Answer from the drawing. Dimensions are ordinates in mm from the lowest x, y and z of the part. Coordinates: 2 decimals unless noted, no trailing zeros. Order: outer loops, then holes, each group sorted by start corner. A loop starts at its lowest first (then second) coordinate and runs counter-clockwise, first axis right, second up. Notation, with made-up numbers: M 2.5,54 L 13.5,54 A32 cw 13.5,92 Z; hole C -0.5,-18 d7. An arc over 180 degrees is marked long. Use a Markdown table: item, result.
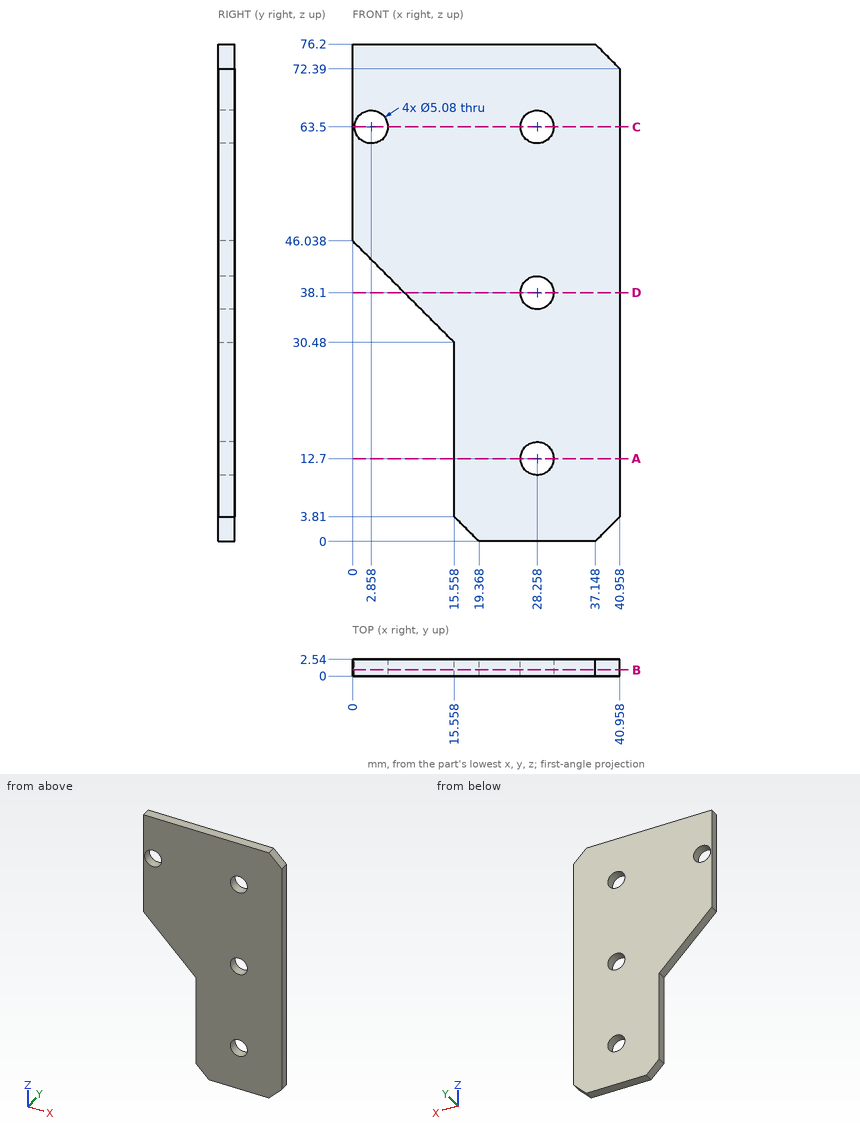
(1) A cutting plane is placed at A-A (z = 12.7). Determine the outline of the cut face in (x, y).
Conclusion:
| item | result |
|---|---|
| outline | M 15.56,0 L 25.72,0 L 25.72,2.54 L 15.56,2.54 Z; M 30.8,0 L 40.96,0 L 40.96,2.54 L 30.8,2.54 Z |
(2) A cutting plane is placed at D-D (z = 38.1). Determine the outline of the cut face in (x, y).
Conclusion:
| item | result |
|---|---|
| outline | M 7.94,0 L 25.72,0 L 25.72,2.54 L 7.94,2.54 Z; M 30.8,0 L 40.96,0 L 40.96,2.54 L 30.8,2.54 Z |
(3) A cutting plane is placed at B-B (y = 0.95). Determine the outline of the cut face in (x, z), then the cut area to 3 significant figures.
Conclusion:
| item | result |
|---|---|
| outline | M 0,46.04 L 15.56,30.48 L 15.56,3.81 L 19.37,0 L 37.15,0 L 40.96,3.81 L 40.96,72.39 L 37.15,76.2 L 0,76.2 Z; hole C 2.86,63.5 d5.08; hole C 28.26,12.7 d5.08; hole C 28.26,38.1 d5.08; hole C 28.26,63.5 d5.08 |
| area | 2,420 mm2 |
(4) Straight lines are drawn through the part: L1, parallel to Z at x = 2.5, y = 2.35 (1 decimal); L2, parallel to Z at x = 2, y = 0.4 (1 decimal); L3, parallel to Z at x = 15.5, y = 1.4 (1 decimal). For each, find the intervals that lie inside material, in ascending order.
Conclusion:
| item | result |
|---|---|
| L1 | 43.5 to 61, 66 to 76.2 |
| L2 | 44 to 61.1, 65.9 to 76.2 |
| L3 | 30.5 to 76.2 |
(5) A cutting plane is placed at C-C (z = 63.5). Determine the outline of the cut face in (x, y).
Conclusion:
| item | result |
|---|---|
| outline | M 0,0 L 0.32,0 L 0.32,2.54 L 0,2.54 Z; M 5.4,0 L 25.72,0 L 25.72,2.54 L 5.4,2.54 Z; M 30.8,0 L 40.96,0 L 40.96,2.54 L 30.8,2.54 Z |
(6) Given P1, Ø1.5, axis at x = 9, y = 1.5, coming from the -Z side; P2, Ø1.3, axis at y = 1.5, z = 23, coming from the -X side, each flat-ended and moving along its own axis, determine where each tip first touches the part or whether it passes through.
Conclusion:
| item | result |
|---|---|
| P1 | z = 36.29 |
| P2 | x = 15.56 |
